```python
from build123d import *

# Parameters (mm, degrees)
SKETCH1_W           = 218
SKETCH1_H           = 117.2
SKETCH1_R           = 1.5
BOSS_EXTRUDE1_DEPTH = 6
SKETCH2_R           = 1.5
CUT_EXTRUDE1_DEPTH  = 6
FILLET1_R           = 7
SKETCH3_W           = 109.333333333
SKETCH3_H           = 59.2
CUT_EXTRUDE2_DEPTH  = 10
FILLET3_R           = 5
CUT_EXTRUDE3_DEPTH  = 10
FILLET4_R           = 5


with BuildPart() as part:
    # Sketch1 → Boss-Extrude1 (new body)
    with BuildSketch(Plane.XY):
        with Locations((-150.609177744, 197.743600407)):
            Rectangle(SKETCH1_W, SKETCH1_H)
        with Locations((-256.109177744, 244.343600407)):
            Circle(SKETCH1_R, mode=Mode.SUBTRACT)
        with Locations((-256.109177744, 151.143600407)):
            Circle(SKETCH1_R, mode=Mode.SUBTRACT)
        with Locations((-45.109177744, 197.743600407)):
            Circle(SKETCH1_R, mode=Mode.SUBTRACT)
        with Locations((-73.109177744, 197.743600407)):
            Circle(SKETCH1_R, mode=Mode.SUBTRACT)
        with Locations((-228.109177744, 244.343600407)):
            Circle(SKETCH1_R, mode=Mode.SUBTRACT)
        with Locations((-228.109177744, 151.143600407)):
            Circle(SKETCH1_R, mode=Mode.SUBTRACT)
    extrude(amount=BOSS_EXTRUDE1_DEPTH)

    # Sketch2 → Cut-Extrude1 (cut)
    with BuildSketch(Plane.XY.offset(6)):
        with Locations((-195.942511077, 151.143600407)):
            Circle(SKETCH2_R)
        with Locations((-177.942511077, 151.143600407)):
            Circle(SKETCH2_R)
        with Locations((-195.942511077, 244.343600407)):
            Circle(SKETCH2_R)
        with Locations((-177.942511077, 244.343600407)):
            Circle(SKETCH2_R)
    extrude(amount=-CUT_EXTRUDE1_DEPTH, mode=Mode.SUBTRACT)

    # Fillet1
    fillet1_edges = [part.edges().sort_by_distance(p)[0] for p in [
        (-259.609177744, 256.343600407, 3),
        (-41.609177744, 256.343600407, 3),
        (-41.609177744, 139.143600407, 3),
        (-259.609177744, 139.143600407, 3),
    ]]
    fillet(fillet1_edges, radius=FILLET1_R)

    # Sketch3 → Cut-Extrude2 (cut)
    with BuildSketch(Plane(origin=(0, 0, 0), x_dir=(-1, 0, 0), z_dir=(0, 0, -1))):
        with Locations((168.942511078, 197.743600407)):
            Rectangle(SKETCH3_W, SKETCH3_H)
    extrude(amount=-CUT_EXTRUDE2_DEPTH, mode=Mode.SUBTRACT)

    # Fillet3
    fillet3_edges = [part.edges().sort_by_distance(p)[0] for p in [
        (-114.275844411, 168.143600407, 3),
        (-114.275844411, 227.343600407, 3),
        (-223.609177744, 227.343600407, 3),
        (-223.609177744, 168.143600407, 3),
    ]]
    fillet(fillet3_edges, radius=FILLET3_R)

    # Sketch4 → Cut-Extrude3 (cut)
    with BuildSketch(Plane(origin=(0, 0, 0), x_dir=(-1, 0, 0), z_dir=(0, 0, -1))):
        Polygon((84.298987117, 241.343600407), (69.597266226, 241.343600407), (69.597266226, 205.418600407), (77.609177744, 205.418600407), (77.609177744, 190.068600407), (69.597266226, 190.068600407), (69.597266226, 154.143600407), (84.298987117, 154.143600407), (104.275844411, 197.743600407), align=None)
    extrude(amount=-CUT_EXTRUDE3_DEPTH, mode=Mode.SUBTRACT)

    # Fillet4
    fillet4_edges = [part.edges().sort_by_distance(p)[0] for p in [
        (-69.597266226, 241.343600407, 3),
        (-84.298987117, 241.343600407, 3),
        (-104.275844411, 197.743600407, 3),
        (-84.298987117, 154.143600407, 3),
        (-69.597266226, 154.143600407, 3),
    ]]
    fillet(fillet4_edges, radius=FILLET4_R)


solid = part.part
```
Source: CAD feature listing. Evaluate the final solid. Frame: model axes, mm. A direction names the side the tool comes from. Give positions to 0.01 mm unless a question says otherwise; leave off trailing zeros. Loops run counter-clockwise (first coordinate to the right, second up) from the corner with the lowest first, then second, coordinate; pieces in that order, holes last. Notation, with made-up numbers: (-15, 89) -> (27, 89) arc R19 cw to (27, 101) -> close; hole circle Ø5 at (-12, 85). An arc over 180 degrees is marked (long way). Use a Markdown table: item, result. Add a question column.
(1) Section query B-B (y = 182.5). Output: boundary loops of the cut face in (x, z).
(2) Ray query, line 1 (X direction, y = 185, z = 3); line 2 (Y direction, x = -75, z = 5.25); line 3 (X direction, y = 211.5, z = 2.25). Return the intervals inside material, ascending.
(3) Section query D-D (z = 3). Count the separate pieces of the cut face and the enclosed holes in it, then the cut area to 3 significant figures.
(4) Section query C-C (y = 162). Output: boundary loops of the cut face in (x, z).
(5) Section query A-A (x = -134.5). Output: boundary loops of the cut face in (y, z), then the cut area to 3 significant figures.
(6) Access query for faces 1 (the face through (-43.714, 254.347, 3.042)), 2 (the face through (-222.106, 225.918, 3.042)). Directions: +Z, -Z, +X, -X, +Y, -Y. A direction counts if a zero-diameter tool reaches every point of the face in a straight line with its end or side. Return the directions, or none.
(7) Pull-direction query (Y, two-part tool) for faces 3 (the face through (-71.023, 239.84, 3.042)), 4 (the face through (-222.183, 169.647, 3.042)), 5 (the face through (-43.714, 141.14, 3.042)), 6 (the face through (-152, 256.344, 3)); classes: +Y half, -Y half, draft (parallel to the pull), parting line (faces both ways), or undercut.
Checked values:
| question | item | result |
|---|---|---|
| 1 | outline | (-259.61, 0) -> (-223.61, 0) -> (-223.61, 6) -> (-259.61, 6) -> close; (-114.28, 0) -> (-97.29, 0) -> (-97.29, 6) -> (-114.28, 6) -> close; (-69.6, 0) -> (-41.61, 0) -> (-41.61, 6) -> (-69.6, 6) -> close |
| 2 | line 1 | -259.61 to -223.61, -114.28 to -98.44, -69.6 to -41.61 |
| 2 | line 2 | 139.14 to 154.14, 190.07 to 205.42, 241.34 to 256.34 |
| 2 | line 3 | -259.61 to -223.61, -114.28 to -97.97, -69.6 to -41.61 |
| 3 | separate pieces | 1 |
| 3 | enclosed holes | 12 |
| 3 | area | 17,000 mm^2 |
| 4 | outline | (-259.61, 0) -> (-87.9, 0) -> (-87.9, 6) -> (-259.61, 6) -> close; (-69.6, 0) -> (-41.61, 0) -> (-41.61, 6) -> (-69.6, 6) -> close |
| 5 | outline | (139.14, 0) -> (168.14, 0) -> (168.14, 6) -> (139.14, 6) -> close; (227.34, 0) -> (256.34, 0) -> (256.34, 6) -> (227.34, 6) -> close |
| 5 | area | 348 mm^2 |
| 6 | face 1 | +Z, -Z, +X, +Y |
| 6 | face 2 | +Z, -Z |
| 7 | face 3 | undercut |
| 7 | face 4 | undercut |
| 7 | face 5 | -Y half |
| 7 | face 6 | +Y half |
